Check sheet for the modelled part. Datum: model origin and axes. Units: mm. A direction names the side the tool comes from. Coordinates: 2 decimals unless noted, no trailing zeros. Write each loop counter-clockwise with the first axis right and the second up, starting at its lowest first coordinate (ties: lowest second). Pieces come first, ordered by that corner, then holes. Notation, with made-up numbers: M -2,46.5 L 49,46.5 A19 ccw 49,75.5 Z; hole C 87,-38.75 d11. An arc over 180 degrees is marked long. Answer as CSV lines item,"result". Start each with the question number.
Q1. Sectioned sample at A-A, the plane z = 0. Record the cut outline in (x, y) (3 decimals), then the cut area to 3 significant figures.
Q2. Depth check by flat-ended pin: pin 1 Ø4 at (y, z) = (15, 7) entering from +X; pin 2 Ø1 at (y, z) = (7.5, -0.5) entering from +X; pin 3 Ø12 at (x, y) = (0.5, 16) entering from -Z. Enter the tip coordinate at first touch or a pass-through.
Q3. Thickness scan on line 1 along X through (y, z) = (16, 0); line 2 along Z through (x, y) = (-6.25, 43.5); line 3 along X through (y, z) = (47, -6.5). Record the ranges inside material, lowest first. Write a range as from..to.
Q4. Sectioned sample at D-D, the plane z = -7.5. Record the cut outline in (x, y), then the cut area to 3 significant figures.
Q5. Access from +Z, -Z, +X, -X, +Y, -Y to the whole of each face (thin tool, end or side, straight path). Record for faces 1 (the flat face through (0, 0, 0)), 2 (the cylindrical face through (-6.3, 23.1, -0.8)), 3 (the flat face through (-2.08, 47.41, -0.15)).
Q6. Sectioned sample at B-B, the plane x = 0. Record the cut outline in (y, z) (3 decimals).
Q7. Mould release check, pull along X, two halves, no side actions. Record for faces 4 (the flat face through (-6, 43.18, -3)), 5 (the cylindrical face through (-3.815, 43.953, 12.114)), 6 (the flat face through (0, 46.052, 0)): pulls with the +X half, pulls with the -X half, needs draft (parallel to the pull), parting line crosses it, or undercut.
Q8. Sectioned sample at C-C, the plane y = 28. Record the cut outline in (x, z).
from build123d import *

# Parameters (mm, degrees)
CUT_EXTRUDE1_DEPTH      = 53.924726322676435
CUT_EXTRUDE1_DEPTH_BACK = 53.924726322676435
CHAMFER1_SIZE           = 2.54


# Read off the part's stored shape, not the designer's step: Dome1
with BuildPart() as part:
    # Sketch1 → Revolve1 (revolve)
    with BuildSketch(Plane.XY, mode=Mode.PRIVATE) as revolve1_sk:
        Polygon((0, 0), (-6.3500000000000005, 0), (-6.3500000000000005, 43.17999999999999), (-12.700000000000003, 43.17999999999999), (-12.700000000000003, 44.70399999999999), (0, 44.70399999999999), align=None)
    revolve(revolve1_sk.sketch.rotate(Axis((0, 0, 0), (0, -1, 0)), 270), axis=Axis((0, 0, 0), (0, -1, 0)))

    # Dome1 outline → Dome1 (revolve)
    with BuildSketch(Plane.XY):
        with BuildLine():
            Line((0, 44.704), (12.700000013, 44.703999987))
            ThreePointArc((12.700000013, 44.703999987), (6.839159314, 48.466898259), (0, 49.784))
            Line((0, 49.784), (0, 44.704))
        make_face()
    revolve(axis=Axis((0, 0, 0), (0, 1, 0)))

    # Sketch2 → Cut-Extrude1 (cut, two sides: drawn at the far end of the back side and taken through both)
    with BuildSketch(Plane.XY.offset(-CUT_EXTRUDE1_DEPTH_BACK)):
        Polygon((-64.2561959287237, 145.90092038345463), (-3.3800930162397096, 49.47113236614868), (-1.2214464709934951, 46.05176386515196), (1.2214464709934951, 46.05176386515196), (3.3800930162397096, 49.47113236614868), (64.2561959287237, 145.90092038345463), (64.2561959287237, 373.97638090364217), (-64.2561959287237, 373.97638090364217), align=None)
    extrude(amount=CUT_EXTRUDE1_DEPTH + CUT_EXTRUDE1_DEPTH_BACK, mode=Mode.SUBTRACT)

    # Chamfer1
    chamfer1_edges = [part.edges().sort_by_distance(p)[0] for p in [
        (-2.19e-15, 0, -6.3500000000000005),
    ]]
    chamfer(chamfer1_edges, length=CHAMFER1_SIZE)


solid = part.part
Output:
1,outline,"M -12.7,43.18 L -6.35,43.18 L -6.35,2.54 L -3.81,0 L 3.81,0 L 6.35,2.54 L 6.35,43.18 L 12.7,43.18 L 12.7,44.704 A18.415 ccw 3.38,49.471 L 1.221,46.052 L -1.221,46.052 L -3.38,49.471 A18.415 ccw -12.7,44.704 Z"
1,area,"652 mm^2"
2,pin 1,"stops at x = 3.91"
2,pin 2,"stops at x = 6.35"
2,pin 3,"stops at z = -6.35"
3,line 1,"x = -6.35..6.35"
3,line 2,"z = -11.06..11.06"
3,line 3,"x = -7.25..-1.82, 1.82..7.25"
4,outline,"M -10.25,43.18 L 10.25,43.18 L 10.25,44.7 A16.82 ccw 2.46,48.01 L 1.22,46.05 L -1.22,46.05 L -2.46,48.01 A16.82 ccw -10.25,44.7 Z"
4,area,"72.1 mm^2"
5,face 1,"+Z, -Z, +X, -X, -Y"
5,face 2,"-Y"
5,face 3,"+Z, -Z, +Y"
6,outline,"M 0,-3.81 L 2.54,-6.35 L 43.18,-6.35 L 43.18,-12.7 L 44.704,-12.7 A18.415 ccw 46.052,-11.114 L 46.052,11.114 A18.415 ccw 44.704,12.7 L 43.18,12.7 L 43.18,6.35 L 2.54,6.35 L 0,3.81 Z"
7,face 4,"needs draft"
7,face 5,"parting line crosses it"
7,face 6,"undercut"
8,outline,"C 0,0 d12.7"
